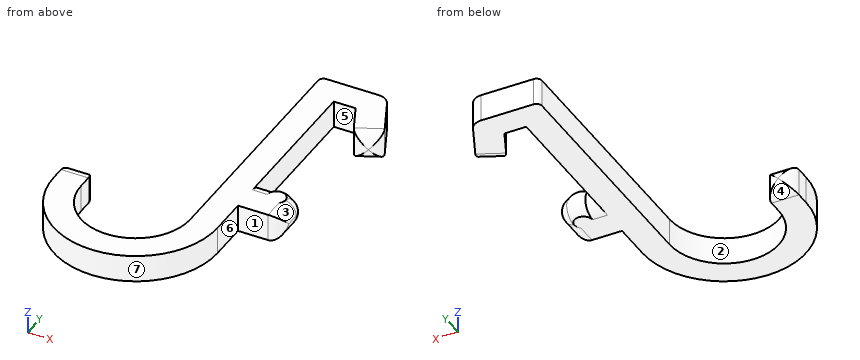
```python
from build123d import *

# Parameters (mm, degrees)
EXTRUDE_1_DEPTH     = 5
FILLET_1_R          = 2.5
FILLET_2_R          = 1
EXTRUDE_2_DEPTH     = 8
FILLET_3_R          = 2.5
SKETCH_5_W          = 1.467751534
SKETCH_5_H          = 4.178210798
SKETCH_5_W_2        = 1.389566385
CUT_EXTRUDE_1_DEPTH = 20


with BuildPart() as part:
    # 草图1 → 凸台-拉伸1 (new body)
    with BuildSketch(Plane.XY):
        with BuildLine():
            Line((0, 0), (0, 28))
            Line((0, 28), (4, 28))
            Line((4, 28), (7.380946094, 20.749537704))
            Line((7.380946094, 20.749537704), (11.912485029, 22.862629012))
            Line((11.912485029, 22.862629012), (7.185351304, 33))
            Line((7.185351304, 33), (-5, 33))
            Line((-5, 33), (-5, -12))
            ThreePointArc((-5, -12), (-15, -22), (-25, -12))
            Line((-25, -12), (-25, -7))
            Line((-25, -7), (-30, -7))
            Line((-30, -7), (-30, -12))
            ThreePointArc((-30, -12), (-15, -27), (0, -12))
            Line((0, -12), (0, -5))
            Line((0, -5), (8, -5))
            Line((8, -5), (8, 0))
            Line((8, 0), (0, 0))
        make_face()
    extrude(amount=EXTRUDE_1_DEPTH)

    # 圆角1
    fillet_1_edges = [part.edges().sort_by_distance(p)[0] for p in [
        (-27.5, -7, 0),
        (9.646715562, 21.806083358, 0),
        (9.646715562, 21.806083358, 5),
        (-30, -7, 2.5),
        (-25, -7, 2.5),
        (7.185351304, 33, 2.5),
        (11.912485029, 22.862629012, 2.5),
        (7.380946094, 20.749537704, 2.5),
        (-27.5, -7, 5),
    ]]
    fillet(fillet_1_edges, radius=FILLET_1_R - 0.0001)  # a hair under: the kernel refuses the full size

    # 圆角2
    fillet_2_edges = [part.edges().sort_by_distance(p)[0] for p in [
        (-5, 33, 2.5),
    ]]
    fillet(fillet_2_edges, radius=FILLET_2_R)

    # 草图3 → 凸台-拉伸2 (add)
    with BuildSketch(Plane(origin=(0, 0, 0), x_dir=(0, 0, -1), z_dir=(1, 0, 0))):
        with BuildLine():
            Line((-5, 0), (0, 0))
            ThreePointArc((0, 0), (-2.5, 2.5), (-5, 0))
        make_face()
    extrude(amount=EXTRUDE_2_DEPTH)

    # 圆角3
    fillet_3_edges = [part.edges().sort_by_distance(p)[0] for p in [
        (8, -2.5, 0),
        (8, -5, 2.5),
        (8, -2.5, 5),
        (8, 2.5, 2.5),
    ]]
    fillet(fillet_3_edges, radius=FILLET_3_R - 0.0001)  # a hair under: the kernel refuses the full size

    # 草图4 → 旋转3 (revolve)
    with BuildSketch(Plane(origin=(4.4, 0, 0), x_dir=(0, 0, -1), z_dir=(1, 0, 0))):
        with BuildLine():
            Line((-5.5, 0), (0.5, 0))
            ThreePointArc((0.5, 0), (-2.5, 3), (-5.5, 0))
        make_face()
    revolve(axis=Axis((4.4, 0, 2.5), (0, 0, -1)))

    # 草图5 → 切除-拉伸1 (cut)
    with BuildSketch(Plane.ZY.offset(5)):
        with Locations((-0.733875767, -0.010051234)):
            Rectangle(SKETCH_5_W, SKETCH_5_H)
        with Locations((5.694783193, -0.010051234)):
            Rectangle(SKETCH_5_W_2, SKETCH_5_H)
    extrude(amount=-CUT_EXTRUDE_1_DEPTH, mode=Mode.SUBTRACT)


solid = part.part
```
Verification items for the finished model (mm, model axes). Face numbers are marked on the shaded views. A direction names the side the tool comes from. Give positions to 0.01 mm unless a question says otherwise; leave off trailing zeros. Loops run counter-clockwise (first coordinate to the right, second up) from the corner with the lowest first, then second, coordinate; pieces in that order, holes last.
1. Thickness scan on line 1 (X direction, y = -11.5, z = 0.5); line 2 (X direction, y = 14, z = 3.85); line 3 (X direction, y = 27, z = 0.65). Record the ranges inside material, lowest first.
2. Section check D-D, the plane y = 5. Enter the section's corners in (x, z), then the cut area to 3 significant figures.
3. Mould release check, pull along X, two halves, no side actions. Record for the marked faces 1, 2 and 3: released by +X, released by -X, zero draft, split by the parting line, or undercut.
4. Section check A-A, the plane y = -8.5. Enter the section's corners in (x, z).
5. Set-up check for the marked faces 4, 5, 6 and 7: record each of +Z, -Z, +X, -X, +Y, -Y from which the full face is reachable in a straight line by a thin tool's end or side.
6. Section check B-B, the plane x = -15. Enter the section's corners in (y, z).
7. Go/stop test with flat-tipped pins: pin 1 Ø2 at (y, z) = (-10.5, 1.5) entering from +X; pin 2 Ø1.5 at (y, z) = (-14.5, 1.5) entering from +X; pin 3 Ø2.5 at (y, z) = (3, 3.5) entering from -X. Record where each tip stops, or that it passes through.
8. Section check C-C, the plane y = -16.5. Enter the section's corners in (x, z).
Geometry says:
1. line 1: x = -30 to -25, -5 to 0
1. line 2: x = -5 to 0
1. line 3: x = -5 to 0, 4.47 to 9.98
2. outline: (-5, 0) - (0, 0) - (0, 5) - (-5, 5) - close
2. area: 25.0 mm2
3. face 1: zero draft
3. face 2: undercut
3. face 3: released by +X
4. outline: (-29.79, 0.21) - (-25.21, 0.21) - (-25.21, 4.79) - (-29.79, 4.79) - close; (-5, 0) - (0, 0) - (0, 5) - (-5, 5) - close
5. face 4: -Z, -X, +Y
5. face 5: +Z, -Z
5. face 6: +Z, -Z, +X, -Y
5. face 7: +Z, -Z, -Y
6. outline: (-27, 0) - (-22, 0) - (-22, 5) - (-27, 5) - close
7. pin 1: stops at x = 0
7. pin 2: stops at x = -0.1
7. pin 3: stops at x = -5
8. outline: (-29.31, 0) - (-23.93, 0) - (-23.93, 5) - (-29.31, 5) - close; (-6.07, 0) - (-0.69, 0) - (-0.69, 5) - (-6.07, 5) - close
